Model file for the job. Use its own axes, mm. A direction names the side the tool comes from. Round coordinates to 2 decimals unless told otherwise and drop trailing zeros. Order: outer loops, then holes, each group sorted by start corner. A loop starts at its lowest first (then second) coordinate and runs counter-clockwise, first axis right, second up. Notation, with made-up numbers: (77, 24) - (97, 24) arc R16 cw to (97, 52) - close; hole circle Ø4 at (-39, -13.75). An arc over 180 degrees is marked (long way). Write item = value, one per line.
```python
from build123d import *

# Parameters (mm, degrees)
SKETCH1_R           = 28.5
BOSS_EXTRUDE1_DEPTH = 6.2
SKETCH2_R           = 14.26
BOSS_EXTRUDE2_DEPTH = 12.7
SKETCH3_R           = 2.75
CUT_EXTRUDE1_DEPTH  = 19.9


with BuildPart() as part:
    # Sketch1 → Boss-Extrude1 (new body)
    with BuildSketch(Plane.XY):
        Circle(SKETCH1_R)
        Polygon((7.332348419, 0), (3.666174209, 6.35), (-3.666174209, 6.35), (-7.332348419, 0), (-3.666174209, -6.35), (3.666174209, -6.35), align=None, mode=Mode.SUBTRACT)
    extrude(amount=BOSS_EXTRUDE1_DEPTH)

    # Sketch2 → Boss-Extrude2 (add)
    with BuildSketch(Plane.XY.offset(6.2)):
        Circle(SKETCH2_R)
        Polygon((3.666174209, -6.35), (7.332348419, 0), (3.666174209, 6.35), (-3.666174209, 6.35), (-7.332348419, 0), (-3.666174209, -6.35), align=None, mode=Mode.SUBTRACT)
    extrude(amount=BOSS_EXTRUDE2_DEPTH)

    # Sketch3 → Cut-Extrude1 (cut, through all)
    with BuildSketch(Plane(origin=(0, 0, 0), x_dir=(-1, 0, 0), z_dir=(0, 0, -1))):
        with Locations((-11.75, 20.351596989)):
            Circle(SKETCH3_R)
        with Locations((11.75, 20.351596989)):
            Circle(SKETCH3_R)
        with Locations((23.5, 0)):
            Circle(SKETCH3_R)
        with Locations((11.75, -20.351596989)):
            Circle(SKETCH3_R)
        with Locations((-11.75, -20.351596989)):
            Circle(SKETCH3_R)
        with Locations((-23.5, 0)):
            Circle(SKETCH3_R)
    extrude(amount=-CUT_EXTRUDE1_DEPTH, mode=Mode.SUBTRACT)


solid = part.part
```
1) Cut at C-C (x = -11.75). Write the cut outline in (y, z).
Conclusion:
outline = (-25.97, 0) - (-23.1, 0) - (-23.1, 6.2) - (-25.97, 6.2) - close; (-17.6, 0) - (17.6, 0) - (17.6, 6.2) - (8.08, 6.2) - (8.08, 18.9) - (-8.08, 18.9) - (-8.08, 6.2) - (-17.6, 6.2) - close; (23.1, 0) - (25.97, 0) - (25.97, 6.2) - (23.1, 6.2) - close
2) Flat gauge pins, fed straight in: pin 1 Ø9 at (x, y) = (-11.75, -20.35) entering from +Z; pin 2 Ø4.5 at (x, y) = (11.75, -20.35) entering from -Z; pin 3 Ø3 at (y, z) = (13.5, 6) entering from -X; pin 4 Ø5 at (y, z) = (-14.5, 16) entering from +X. Where does each tip first touch, or does it go through?
Conclusion:
pin_1 = 6.2
pin_2 = through
pin_3 = -25.85
pin_4 = 7.7
3) Cut at D-D (z = 16.75). Write the cut outline in (x, y).
Conclusion:
outline = circle Ø28.52 at (0, 0); hole (-7.33, 0) - (-3.67, -6.35) - (3.67, -6.35) - (7.33, 0) - (3.67, 6.35) - (-3.67, 6.35) - close
4) Cut at A-A (x = 0). Write the cut outline in (y, z), and give its area (3 significant figures).
Conclusion:
outline = (-28.5, 0) - (-6.35, 0) - (-6.35, 18.9) - (-14.26, 18.9) - (-14.26, 6.2) - (-28.5, 6.2) - close; (6.35, 0) - (28.5, 0) - (28.5, 6.2) - (14.26, 6.2) - (14.26, 18.9) - (6.35, 18.9) - close
area = 476 mm^2
5) 3-axis set-ups, long thin cutter, end or side, ignore diameter. For faces 1 (the face through (-5.525, -3.131, 9.318)), 2 (the face through (-7, 13, 6.2)), 3 (the face through (0, 7, 18.9)): which of +Z, -Z, +X, -X, +Y, -Y reach the whole face in a straight line?
Conclusion:
face_1 = +Z, -Z
face_2 = +Z
face_3 = +Z, +X, -X, +Y, -Y
6) Mould opens along X. For faces 4 (the face through (13.601, 4.283, 12.461)), 5 (the face through (0, 7, 0)), 6 (the face through (5.525, 3.131, 9.318)) say: +X half, -X half, draft (parallel to the pull), parting line (faces both ways), or undercut.
Conclusion:
face_4 = parting line
face_5 = draft
face_6 = undercut
7) Wall check: line 1 along Y through (x, z) = (-12.5, 5); line 2 along Y through (x, z) = (-11.75, 2.5); line 3 along X through (y, z) = (21.5, 5.25). Give the ranges that are in metal, low to high.
Conclusion:
line_1 = -25.61 to -23, -17.71 to 17.71, 23 to 25.61
line_2 = -25.97 to -23.1, -17.6 to 17.6, 23.1 to 25.97
line_3 = -18.71 to -14.25, -9.25 to 9.25, 14.25 to 18.71
8) Cut at B-B (z = 5.25). Write the cut outline in (x, y), and give its area (3 significant figures).
Conclusion:
outline = circle Ø57 at (0, 0); hole circle Ø5.5 at (-23.5, 0); hole circle Ø5.5 at (-11.75, -20.35); hole circle Ø5.5 at (-11.75, 20.35); hole (-7.33, 0) - (-3.67, -6.35) - (3.67, -6.35) - (7.33, 0) - (3.67, 6.35) - (-3.67, 6.35) - close; hole circle Ø5.5 at (11.75, -20.35); hole circle Ø5.5 at (11.75, 20.35); hole circle Ø5.5 at (23.5, 0)
area = 2,270 mm^2
